from build123d import *

# Parameters (mm, degrees)
SKETCH1_R                      = 57.15
SEAL_SEAT_HIEGHT_DEPTH         = 5.5372
SKETCH2_R                      = 57.15
SEAL_DIAPHRAM_HIEGHT_DEPTH     = 15.875
SEAL_START                     = 2
SKETCH3_R                      = 57.15
SEAL_SHOULDER_HIEGHT_DEPTH     = 2
SKETCH5_R                      = 11.1125
SEAL_SEAT_FIT_DEPTH            = 5.5372
SKETCH7_R                      = 5.7625
SHAFT_CLEARANCE_DEPTH          = 2
M8_CLEARANCE_HOLE1_D           = 8.4
F_1_4_0_25_PRESS_DOWEL_HOLE1_D = 6.35
SKETCH6_R                      = 12.7
CUT_EXTRUDE1_DEPTH             = 15.875


with BuildPart() as part:
    # Sketch1 → seal seat hieght (new body)
    with BuildSketch(Plane(origin=(0, 0, 0), x_dir=(1, 0, 0), z_dir=(0, 1, 0))):
        with Locations(Location((0, 0, 0), (0, 0, 270))):
            Circle(SKETCH1_R)
    extrude(amount=-SEAL_SEAT_HIEGHT_DEPTH)

    # Sketch2 → seal diaphram hieght (add)
    with BuildSketch(Plane.XZ.offset(5.5372)):
        with Locations(Location((0, 0, 0), (0, 0, 90))):
            Circle(SKETCH2_R)
    extrude(amount=SEAL_DIAPHRAM_HIEGHT_DEPTH)

    # Sketch3 → seal shoulder hieght (add)
    with BuildSketch(Plane(origin=(0, 0, 0), x_dir=(1, 0, 0), z_dir=(0, 1, 0)).offset(SEAL_START)):
        with Locations(Location((0, 0, 0), (0, 0, 270))):
            Circle(SKETCH3_R)
    extrude(amount=-SEAL_SHOULDER_HIEGHT_DEPTH)

    # Sketch5 → seal seat fit (cut)
    with BuildSketch(Plane(origin=(0, 0, 0), x_dir=(1, 0, 0), z_dir=(0, 1, 0))):
        with Locations(Location((0, 0, 0), (0, 0, 270))):
            Circle(SKETCH5_R)
    extrude(amount=-SEAL_SEAT_FIT_DEPTH, mode=Mode.SUBTRACT)

    # Sketch7 → shaft clearance (cut)
    with BuildSketch(Plane(origin=(0, 0, 0), x_dir=(1, 0, 0), z_dir=(0, 1, 0))):
        with Locations(Location((0, 0, 0), (0, 0, 270))):
            Circle(SKETCH7_R)
    extrude(amount=SHAFT_CLEARANCE_DEPTH, mode=Mode.SUBTRACT)

    # M8 Clearance Hole1 (through all)
    with Locations(Plane(origin=(0, 2, 0), x_dir=(1, 0, 0), z_dir=(0, 1, 0))):
        with Locations((-44.45, 0), (0, 44.45), (44.45, 0), (0, -44.45)):
            Hole(M8_CLEARANCE_HOLE1_D / 2)

    # 1/4 (0.25) Press Dowel Hole1 (through all)
    with Locations(Plane(origin=(0, 2, 0), x_dir=(1, 0, 0), z_dir=(0, 1, 0))):
        with Locations((31.430896424, 31.430896424), (-31.430896424, -31.430896424)):
            Hole(F_1_4_0_25_PRESS_DOWEL_HOLE1_D / 2)

    # Sketch6 → Cut-Extrude1 (cut)
    with BuildSketch(Plane(origin=(0, -21.4122, 0), x_dir=(-1, 0, 0), z_dir=(0, -1, 0))):
        with Locations(Location((0, 0, 0), (0, 0, 90))):
            Circle(SKETCH6_R)
    extrude(amount=-CUT_EXTRUDE1_DEPTH, mode=Mode.SUBTRACT)


solid = part.part
The model under review builds one solid part; all positions refer to its coordinate system, in mm. A direction names the side the tool comes from. Give positions to 0.01 mm unless a question says otherwise; leave off trailing zeros. Loops run counter-clockwise (first coordinate to the right, second up) from the corner with the lowest first, then second, coordinate; pieces in that order, holes last. Notation, with made-up numbers: (7.25, 77.25) -> (62.25, 77.25) arc R21 cw to (62.25, 110.25) -> close; hole circle Ø9 at (32, 3.25). An arc over 180 degrees is marked (long way). Put each result on its own line as item: value. Start each with the question number.
1. We need section C-C on y = -3.25. State how many separate pieces and enclosed holes the cut face has, then the cut area to 3 significant figures.
2. Mouldability with a two-part tool opening along X and no side actions: class faces 1 (the face through (2.513, -9.542, -57.095)), 2 (the face through (1.731, 0.986, 5.496)), 3 (the face through (-1, -21.412, -14)) as released by +X, released by -X, zero draft, split by the parting line, or undercut.
3. Wall thickness on probe 1 along X at (y, z) = (-13.75, -1.5); probe 2 along X at (y, z) = (-5, 2.5); probe 3 along Z at (x, y) = (44.45, -10.25): over which ranges is each line inside the solid? List them lowest first.
4. Clearance check with flat-ended pins moving along their axes: P1, Ø8, axis at x = -24.5, y = -8, coming from the +Z side; P2, Ø2, axis at y = -3.5, z = -2.5, coming from the -X side; P3, Ø5, axis at x = 23.5, y = -2.5, coming from the +Z side; P4, Ø10.5, axis at x = 0, z = 0, coming from the -Y side. State where each tip first meets the part, or that it passes through.
5. We need section B-B on x = -44.45. State the section outline as (y, z) points.
6. We need section D-D on z = -44.45. State the section outline as (x, y) points.
7. For faces 4 (the face through (-11.23, -5.537, -0.88)), 5 (the face through (29.97, -9.87, -28.61)), list the 3-axis set-ups (+Z, -Z, +X, -X, +Y, -Y) from which the entire face can be reached by the end or side of a thin tool; tool diameter is ignored.
8. We need section A-A on z = 0. State the section outline as (x, y) points, then the cut area to 3 significant figures.
Determined:
1. separate pieces: 1
1. enclosed holes: 7
1. area: 9,590 mm^2
2. face 1: split by the parting line
2. face 2: undercut
2. face 3: zero draft
3. probe 1: -57.13 to -48.37, -40.53 to -12.61, 12.61 to 40.53, 48.37 to 57.13
3. probe 2: -57.1 to -47.82, -41.08 to -10.83, 10.83 to 41.08, 47.82 to 57.1
3. probe 3: -35.92 to -4.2, 4.2 to 35.92
4. P1: z = 53.35
4. P2: x = -57.13
4. P3: z = 53.15
4. P4: through
5. outline: (-21.41, -35.92) -> (2, -35.92) -> (2, -4.2) -> (-21.41, -4.2) -> close; (-21.41, 4.2) -> (2, 4.2) -> (2, 35.92) -> (-21.41, 35.92) -> close
6. outline: (-35.92, -21.41) -> (-4.2, -21.41) -> (-4.2, 2) -> (-35.92, 2) -> close; (4.2, -21.41) -> (35.92, -21.41) -> (35.92, 2) -> (4.2, 2) -> close
7. face 4: -Y
7. face 5: +Y, -Y
8. outline: (-57.15, -21.41) -> (-48.65, -21.41) -> (-48.65, 2) -> (-57.15, 2) -> close; (-40.25, -21.41) -> (-12.7, -21.41) -> (-12.7, -5.54) -> (-11.11, -5.54) -> (-11.11, 0) -> (-5.76, 0) -> (-5.76, 2) -> (-40.25, 2) -> close; (5.76, 0) -> (11.11, 0) -> (11.11, -5.54) -> (12.7, -5.54) -> (12.7, -21.41) -> (40.25, -21.41) -> (40.25, 2) -> (5.76, 2) -> close; (48.65, -21.41) -> (57.15, -21.41) -> (57.15, 2) -> (48.65, 2) -> close
8. area: 1,730 mm^2
